Could you check a few things on this model? Use its own coordinates, in mm. Face numbers are marked on the shaded views. A direction names the side the tool comes from. Coordinates: 2 decimals unless noted, no trailing zeros. Loops run counter-clockwise (first coordinate to the right, second up) from the corner with the lowest first, then second, coordinate; pieces in that order, holes last. Notation, with made-up numbers: M -23,-10 L -13,-10 A33 cw -13,25 Z; hole C 28.25,80.25 d7. An arc over 180 degrees is marked long. Write each question's results on one line, items separated by ' | '.
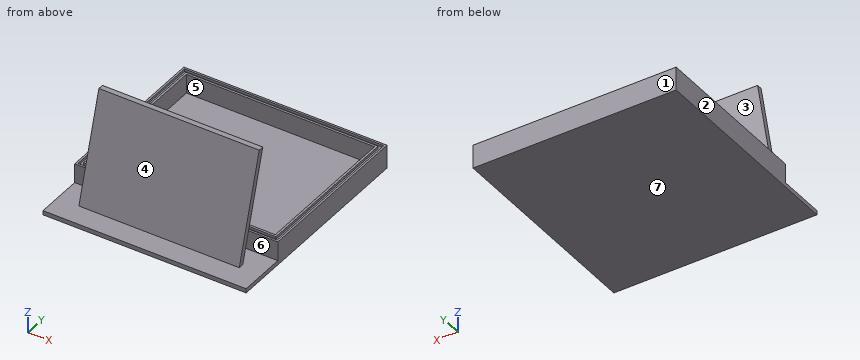
```python
from build123d import *

# Parameters (mm, degrees)
F_190_X_200_TRAY_FLOOR_SKETCH_W                  = 190
F_190_X_200_TRAY_FLOOR_SKETCH_H                  = 200
F_4_MM_TRAY_FLOOR_DEPTH                          = 4
ELECTRONICS_COMPARTMENT_WALL_SKETCH_W            = 190
ELECTRONICS_COMPARTMENT_WALL_SKETCH_H            = 155
ELECTRONICS_COMPARTMENT_WALL_SKETCH_W_2          = 176
ELECTRONICS_COMPARTMENT_WALL_SKETCH_H_2          = 141
F_22_MM_PERIMETER_WALLS_DEPTH                    = 22
F_3_2_START                                      = 22
F_3_MM_CORD_GASKET_GROOVE_SKETCH_W               = 186.4
F_3_MM_CORD_GASKET_GROOVE_SKETCH_H               = 151.4
F_3_MM_CORD_GASKET_GROOVE_SKETCH_W_2             = 180
F_3_MM_CORD_GASKET_GROOVE_SKETCH_H_2             = 145
F_3_2_X_2_3_MM_PERIMETER_GASKET_GROOVE_DEPTH     = 2.3
F_150_MM_WIDE_ANGLED_DISPLAY_BULKHEAD_DEPTH      = 75
F_150_MM_WIDE_ANGLED_DISPLAY_BULKHEAD_DEPTH_BACK = 75


with BuildPart() as part:
    # 190 x 200 Tray Floor Sketch → 4 mm Tray Floor (new body)
    with BuildSketch(Plane.XY):
        with Locations((0, 100)):
            Rectangle(F_190_X_200_TRAY_FLOOR_SKETCH_W, F_190_X_200_TRAY_FLOOR_SKETCH_H)
    extrude(amount=F_4_MM_TRAY_FLOOR_DEPTH)

    # Electronics Compartment Wall Sketch → 22 mm Perimeter Walls (add)
    with BuildSketch(Plane.XY):
        with Locations((0, 122.5)):
            Rectangle(ELECTRONICS_COMPARTMENT_WALL_SKETCH_W, ELECTRONICS_COMPARTMENT_WALL_SKETCH_H)
        with Locations((0, 122.5)):
            Rectangle(ELECTRONICS_COMPARTMENT_WALL_SKETCH_W_2, ELECTRONICS_COMPARTMENT_WALL_SKETCH_H_2, mode=Mode.SUBTRACT)
    extrude(amount=F_22_MM_PERIMETER_WALLS_DEPTH)

    # 3 mm Cord Gasket Groove Sketch → 3.2 x 2.3 mm Perimeter Gasket Groove (cut)
    with BuildSketch(Plane.XY.offset(F_3_2_START)):
        with Locations((0, 122.5)):
            Rectangle(F_3_MM_CORD_GASKET_GROOVE_SKETCH_W, F_3_MM_CORD_GASKET_GROOVE_SKETCH_H)
        with Locations((0, 122.5)):
            Rectangle(F_3_MM_CORD_GASKET_GROOVE_SKETCH_W_2, F_3_MM_CORD_GASKET_GROOVE_SKETCH_H_2, mode=Mode.SUBTRACT)
    extrude(amount=-F_3_2_X_2_3_MM_PERIMETER_GASKET_GROOVE_DEPTH, mode=Mode.SUBTRACT)

    # Angled Display Bulkhead Side Profile → 150 mm Wide Angled Display Bulkhead (add, two sides: drawn at the far end of the back side and taken through both)
    with BuildSketch(Plane(origin=(0, 0, 0), x_dir=(0, 0, -1), z_dir=(1, 0, 0)).offset(-F_150_MM_WIDE_ANGLED_DISPLAY_BULKHEAD_DEPTH_BACK)):
        Polygon((-2, 20), (-2, 25), (-100, 54), (-100, 49), align=None)
    extrude(amount=F_150_MM_WIDE_ANGLED_DISPLAY_BULKHEAD_DEPTH + F_150_MM_WIDE_ANGLED_DISPLAY_BULKHEAD_DEPTH_BACK)


solid = part.part
```
(1) Imagine slicing it at C-C, the plane y = 36.5. List the corners of the cut face in (x, z) for me, and give its area (3 significant figures).
Reported:
outline: M -95,0 L 95,0 L 95,4 L -95,4 Z; M -75,40.86 L 75,40.86 L 75,57.76 L -75,57.76 Z | area: 3,290 mm2
(2) Please list where these lines run through material, in increasing order: probe 1 along X at (y, z) = (155, 20.5); probe 2 along X at (y, z) = (149.5, 14); probe 3 along Y at (x, z) = (-51, 11). Write a range as from..to.
Reported:
probe 1: x = -95..-93.2, -90..-88, 88..90, 93.2..95 | probe 2: x = -95..-88, 88..95 | probe 3: y = 22.66..27.66, 45..52, 193..200
(3) Imagine slicing it at D-D, the plane x = -80.5. List the corners of the cut face in (y, z) for me, and give its area (3 significant figures).
Reported:
outline: M 0,0 L 200,0 L 200,22 L 198.2,22 L 198.2,19.7 L 195,19.7 L 195,22 L 193,22 L 193,4 L 52,4 L 52,22 L 50,22 L 50,19.7 L 46.8,19.7 L 46.8,22 L 45,22 L 45,4 L 0,4 Z | area: 1,040 mm2
(4) Will these pins go through, and if not, where does the flat tip stop? P1, Ø1.2, axis at x = -28, z = 20.5, coming from the -Y side; P2, Ø9, axis at x = 0, z = 17.5, coming from the -Y side; P3, Ø5.5, axis at x = 16, z = 14, coming from the -Y side; P4, Ø8, axis at x = -52.5, y = 176, coming from the -Z side.
Reported:
P1: stops at y = 25.3 | P2: stops at y = 23.26 | P3: stops at y = 22.74 | P4: stops at z = 0
(5) Which directions (+Z, -Z, +X, -X, +Y, -Y) give clear straight access to the entire face, cutting with the end or side of a thin tool? Please do the marked faces 5, 6 and 7.
Reported:
face 5: +Z | face 6: +X, -X | face 7: -Z, +X, -X, +Y, -Y
(6) Imagine slicing it at A-A, the plane y = 156. List the corners of the cut face in (x, z) for me.
Reported:
outline: M -95,0 L 95,0 L 95,22 L 93.2,22 L 93.2,19.7 L 90,19.7 L 90,22 L 88,22 L 88,4 L -88,4 L -88,22 L -90,22 L -90,19.7 L -93.2,19.7 L -93.2,22 L -95,22 Z
(7) If we mould it in two halves opening along Y, with no side actions, what happens to the marked faces 1, 2, 3 and 4? For each: released by +Y, released by -Y, zero draft, split by the parting line, or undercut.
Reported:
face 1: released by +Y | face 2: zero draft | face 3: undercut | face 4: released by -Y
(8) Imagine slicing it at B-B, the plane x = 15.5. List the corners of the cut face in (y, z) for me, and give its area (3 significant figures).
Reported:
outline: M 0,0 L 200,0 L 200,22 L 198.2,22 L 198.2,19.7 L 195,19.7 L 195,22 L 193,22 L 193,4 L 52,4 L 52,22 L 50,22 L 50,19.7 L 46.8,19.7 L 46.8,22 L 45,22 L 45,4 L 25.59,4 L 54,100 L 49,100 L 20.59,4 L 0,4 Z | area: 1,520 mm2
